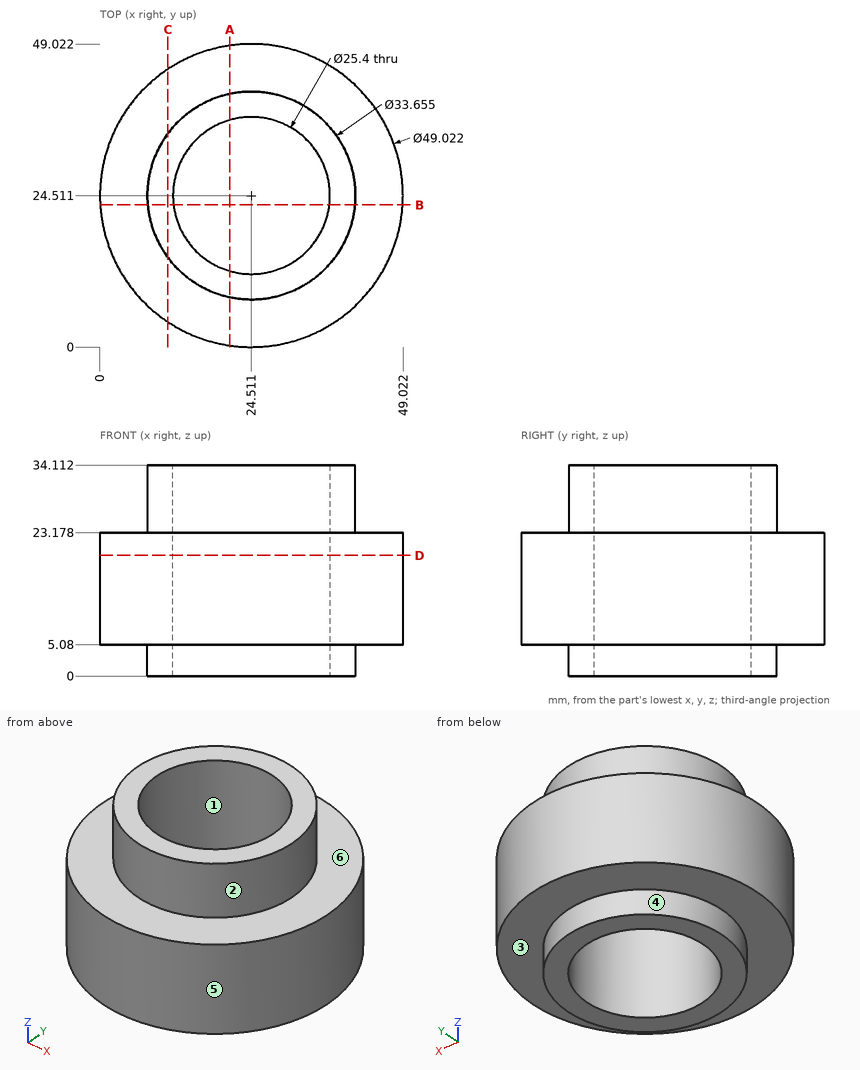
Input: dimensioned drawing with shaded views. Units: mm. Origin: part minimum x, y, z. A direction names the side the tool comes from. Give positions to 0.01 mm unless a question says otherwise; leave off trailing zeros. Write each loop counter-clockwise with the first axis right and the second up, starting at its lowest first coordinate (ties: lowest second). Pieces come first, ordered by that corner, then holes. Notation, with made-up numbers: (-12, 64.25) -> (39, 64.25) arc R18 cw to (39, 95.25) -> close; hole circle Ø7 at (17, 45.25). An arc over 180 degrees is marked (long way). Return JSON: item names as keys, results as strings. Group by question number.
1. Section C-C, the plane x = 11. Output: boundary loops of the cut face in (y, z), then the cut area to 3 significant figures.
2. Pin query (flat end, axial travel): pin 1 Ø10 at (x, z) = (34, 23) entering from +Y; pin 2 Ø6 at (x, z) = (30, 5.5) entering from +Y (1 decimal); pin 3 Ø1 at (y, z) = (40.5, 6.5) entering from +X. Return the tip coordinate at first contact, or that it passes through.
3. Section D-D, the plane z = 19.5. Output: boundary loops of the cut face in (x, y).
4. Access query for the marked faces 4, 5 and 6. Directions: +Z, -Z, +X, -X, +Y, -Y. A direction counts if a zero-diameter tool reaches every point of the face in a straight line with its end or side. Return the directions, or none.
5. Material intervals for line 1 (Z direction, x = 3, y = 35); line 2 (Y direction, x = 29.5, z = 14); line 3 (Y direction, x = 33, z = 32) (1 decimal), sorted ascending. Write a range as from..to.
6. Section B-B, the plane y = 23. Output: boundary loops of the cut face in (x, z) (1 decimal).
7. Section A-A, the plane x = 21. Output: boundary loops of the cut face in (y, z) (1 decimal).
8. Mould query, pull axis X, two halves, no side actions, for the marked faces 1, 2 and 3. Classes: +X half, -X half, draft (parallel to the pull), parting line (faces both ways), or undercut.
Determined:
{
 "1": {"outline": "(4.06, 5.08) -> (14.48, 5.08) -> (14.48, 0) -> (34.54, 0) -> (34.54, 5.08) -> (44.96, 5.08) -> (44.96, 23.18) -> (34.54, 23.18) -> (34.54, 34.11) -> (14.48, 34.11) -> (14.48, 23.18) -> (4.06, 23.18) -> close", "area": "1,060 mm2"},
 "2": {"pin 1": "stops at y = 48.61", "pin 2": "stops at y = 48.9", "pin 3": "stops at x = 43.51"},
 "3": {"outline": "circle Ø49.02 at (24.51, 24.51); hole circle Ø25.4 at (24.51, 24.51)"},
 "4": {"face 4": "-Z", "face 5": "+Z, -Z", "face 6": "+Z"},
 "5": {"line 1": "z = 5.08..23.18", "line 2": "y = 0.51..12.83, 36.19..48.51", "line 3": "y = 10..15.1, 34..39"},
 "6": {"outline": "(0, 5.1) -> (7.8, 5.1) -> (7.8, 0) -> (11.9, 0) -> (11.9, 34.1) -> (7.8, 34.1) -> (7.8, 23.2) -> (0, 23.2) -> close; (37.1, 0) -> (41.3, 0) -> (41.3, 5.1) -> (49, 5.1) -> (49, 23.2) -> (41.3, 23.2) -> (41.3, 34.1) -> (37.1, 34.1) -> close"},
 "7": {"outline": "(0.3, 5.1) -> (8.1, 5.1) -> (8.1, 0) -> (12.3, 0) -> (12.3, 34.1) -> (8.1, 34.1) -> (8.1, 23.2) -> (0.3, 23.2) -> close; (36.7, 0) -> (41, 0) -> (41, 5.1) -> (48.8, 5.1) -> (48.8, 23.2) -> (41, 23.2) -> (41, 34.1) -> (36.7, 34.1) -> close"},
 "8": {"face 1": "undercut", "face 2": "parting line", "face 3": "draft"}
}
